Can you work these out from the drawing? Everything is in mm from the part's minimum corner. Coordinates: 2 decimals unless noted, no trailing zeros. Loops run counter-clockwise (first coordinate to the right, second up) from the corner with the lowest first, then second, coordinate; pieces in that order, holes last. Notation, with made-up numbers: (52, 41.5) - (80, 41.5) arc R9 cw to (80, 47.5) - close; hole circle Ø5 at (-20, -28). An arc over 180 degrees is marked (long way). Use CSV: the item, a comma, the result in double quotes.
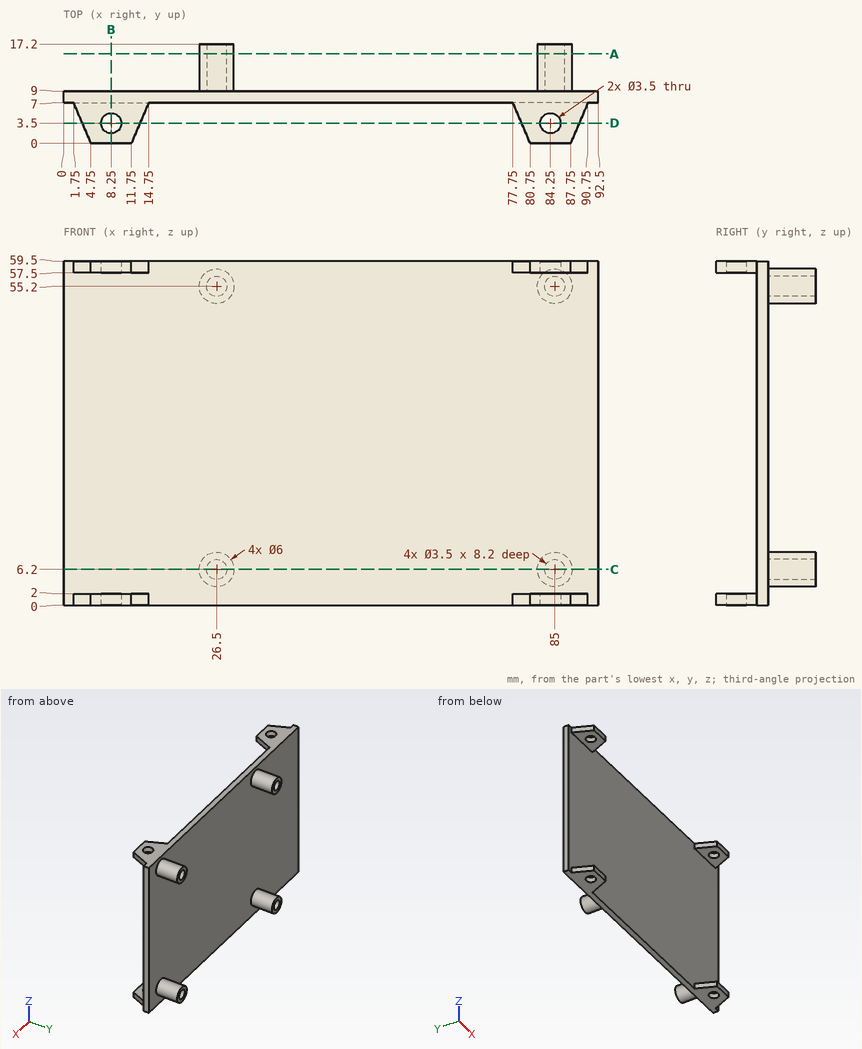
(1) Suppose I cut it at C-C (z = 6.2). Write out the boundary of the cut face in (x, y).
Computed:
outline,"(0, 7) - (92.5, 7) - (92.5, 9) - (88, 9) - (88, 17.2) - (86.75, 17.2) - (86.75, 9) - (83.25, 9) - (83.25, 17.2) - (82, 17.2) - (82, 9) - (29.5, 9) - (29.5, 17.2) - (28.25, 17.2) - (28.25, 9) - (24.75, 9) - (24.75, 17.2) - (23.5, 17.2) - (23.5, 9) - (0, 9) - close"
(2) Suppose I cut it at B-B (x = 8.25). Write out the boundary of the cut face in (y, z), plus the area to 3 significant figures.
Computed:
outline,"(0, 0) - (1.75, 0) - (1.75, 2) - (0, 2) - close; (0, 57.5) - (1.75, 57.5) - (1.75, 59.5) - (0, 59.5) - close; (5.25, 0) - (9, 0) - (9, 59.5) - (5.25, 59.5) - (5.25, 57.5) - (7, 57.5) - (7, 2) - (5.25, 2) - close"
area,"133 mm²"
(3) Suppose I cut it at A-A (y = 15.5). Write out the boundary of the cut face in (x, z).
Computed:
outline,"circle Ø6 at (26.5, 6.2); circle Ø6 at (26.5, 55.2); circle Ø6 at (85, 6.2); circle Ø6 at (85, 55.2); hole circle Ø3.5 at (26.5, 6.2); hole circle Ø3.5 at (26.5, 55.2); hole circle Ø3.5 at (85, 6.2); hole circle Ø3.5 at (85, 55.2)"
(4) Suppose I cut it at D-D (y = 3.5). State how many separate pieces and enclosed holes the cut face has, plus the area to 3 significant figures.
Computed:
separate pieces,"8"
enclosed holes,"0"
area,"52.0 mm²"
(5) Will these pins go through, and if not, where does the flat tip stop? pin 1 (18 mm diameter, centred on x = 46, z = 36.5, fed in from +Y); pin 2 (2 mm diameter, centred on x = 85, z = 55.2, fed in from -Y).
Computed:
pin 1,"stops at y = 9"
pin 2,"stops at y = 7"
(6) Please list where these lines run through material, in increasing order: line 1 (Z direction, x = 85, y = 11.5); line 2 (Y direction, x = 8, z = 1); line 3 (Y direction, x = 22.5, z = 46).
Computed:
line 1,"z = 3.2 to 4.45, 7.95 to 9.2, 52.2 to 53.45, 56.95 to 58.2"
line 2,"y = 0 to 1.77, 5.23 to 9"
line 3,"y = 7 to 9"
